Part model, mm, in its own coordinate system. Face numbers are marked on the shaded views. A direction names the side the tool comes from. Round coordinates to 2 decimals unless told otherwise and drop trailing zeros. Write each loop counter-clockwise with the first axis right and the second up, starting at its lowest first coordinate (ties: lowest second). Pieces come first, ordered by that corner, then holes. Notation, with made-up numbers: (28.5, 49) -> (37.5, 49) arc R19 ccw to (37.5, 83) -> close; hole circle Ø2 at (-17.5, 57). An arc over 180 degrees is marked (long way). Use CSV: the item, a comma, the result in double quotes. Start each with the question number.
(1) Probe line 1 (Y direction, x = -10.5, z = 0.45); line 2 (X direction, y = -1.5, z = 3.5); line 3 (Z direction, x = -9, y = 4). List the from-to ranges inside material, lowest first. Write a range as [from, to].
(2) Drop flat-ended pins along their axis: pin 1 (4 mm diameter, centred on x = -7, z = 2, fed in from +Y); pin 2 (2.5 mm diameter, centred on y = -1, z = 2.5, fed in from -X); pin 3 (1 mm diameter, centred on x = -11.5, y = -3, fed in from +Z); pin 4 (8 mm diameter, centred on x = -2, z = 12.5, fed in from +Y). Give the stop position or say it passes through.
(3) Saw through at B-B (z = 7). Give the cut face in (x, y).
(4) Which spindle directions (+Z, -Z, +X, -X, +Y, -Y) get a long thin tool onto all of the face, cutting with end or side? Do the marked faces 4, 5, 6 and 7. Say none if no direction does.
(5) Two-plate mould, pull along Y, no slides. Class the marked faces 1, 2 and 3: released by +Y, released by -Y, zero draft, split by the parting line, or undercut.
(6) Saw through at A-A (x = 10.5). Count the separate pieces of the cut face and the enclosed holes in it, plus the area to 3 significant figures.
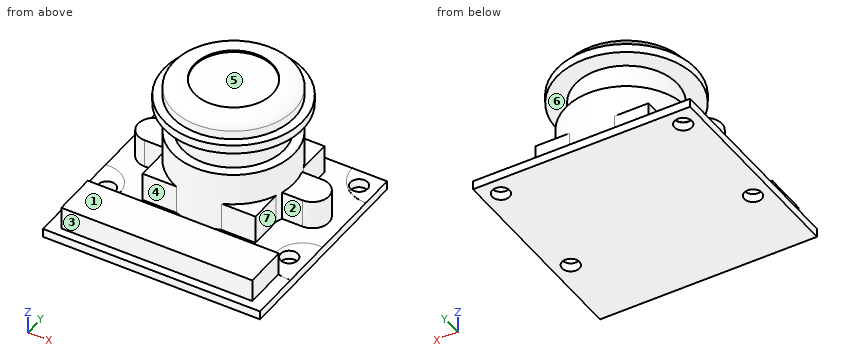
```python
from build123d import *

# Parameters (mm, degrees)
CROQUIS1_W              = 25
CROQUIS1_H              = 24
SALIENTE_EXTRUIR1_DEPTH = 1
CROQUIS2_W              = 22
CROQUIS2_H              = 5
SALIENTE_EXTRUIR2_DEPTH = 2.6
SALIENTE_EXTRUIR3_DEPTH = 3.3
CROQUIS5_R              = 7
SALIENTE_EXTRUIR4_DEPTH = 7
CROQUIS6_R              = 5.85
SALIENTE_EXTRUIR5_DEPTH = 3.5
CROQUIS9_R              = 1
CORTAR_EXTRUIR1_DEPTH   = 1
SALIENTE_EXTRUIR6_START = 0.01
CROQUIS10_R             = 0.972515087
CROQUIS10_R_2           = 1
SALIENTE_EXTRUIR6_DEPTH = 0.01


with BuildPart() as part:
    # Croquis1 → Saliente-Extruir1 (new body)
    with BuildSketch(Plane.XY):
        Rectangle(CROQUIS1_W, CROQUIS1_H)
    extrude(amount=SALIENTE_EXTRUIR1_DEPTH)

    # Croquis2 → Saliente-Extruir2 (add)
    with BuildSketch(Plane.XY.offset(1)):
        with Locations((0, -8.5)):
            Rectangle(CROQUIS2_W, CROQUIS2_H)
    extrude(amount=SALIENTE_EXTRUIR2_DEPTH)

    # Croquis3 → Saliente-Extruir3 (add)
    with BuildSketch(Plane.XY.offset(1)):
        with BuildLine():
            Line((-9.1, 5.4), (-6.5, 5.4))
            Line((-6.5, 5.4), (-6.5, 10))
            Line((-6.5, 10), (6.5, 10))
            Line((6.5, 10), (6.5, 5.4))
            Line((6.5, 5.4), (9.1, 5.4))
            ThreePointArc((9.1, 5.4), (11, 3.5), (9.1, 1.6))
            Line((9.1, 1.6), (6.5, 1.6))
            Line((6.5, 1.6), (6.5, -3))
            Line((6.5, -3), (-6.5, -3))
            Line((-6.5, -3), (-6.5, 1.6))
            Line((-6.5, 1.6), (-9.1, 1.6))
            ThreePointArc((-9.1, 1.6), (-11, 3.5), (-9.1, 5.4))
        make_face()
    extrude(amount=SALIENTE_EXTRUIR3_DEPTH)

    # Croquis5 → Saliente-Extruir4 (add)
    with BuildSketch(Plane.XY.offset(1)):
        with Locations(Location((0, 3.5, 0), (0, 0, 164.250707132))):
            Circle(CROQUIS5_R)
    extrude(amount=SALIENTE_EXTRUIR4_DEPTH)

    # Croquis6 → Saliente-Extruir5 (add)
    with BuildSketch(Plane.XY.offset(8)):
        with Locations((0, 3.5)):
            Circle(CROQUIS6_R)
    extrude(amount=SALIENTE_EXTRUIR5_DEPTH)

    # Croquis8 → Revolución1 (revolve)
    with BuildSketch(Plane(origin=(0, 3.5, 0), x_dir=(-1, 0, 0), z_dir=(0, -1, 0)), mode=Mode.PRIVATE) as revoluci_n1_sk:
        with BuildLine():
            Line((0, -11.5), (-8, -11.5))
            Line((-8, -11.5), (-8, -12.5))
            Line((-8, -12.5), (-7, -12.5))
            Line((-7, -12.5), (-7, -13.5))
            add(Edge.make_bspline(
                [(-7, -13.5), (-7, -14.5), (-4.5, -14.5)],
                knots=[0, 0, 0, 1.570796327, 1.570796327, 1.570796327], degree=2, weights=[1, 0.707106781, 1]))
            Line((-4.5, -14.5), (-4.5, -14.3))
            Line((-4.5, -14.3), (0, -14.3))
            Line((0, -14.3), (0, -11.5))
        make_face()
    revolve(revoluci_n1_sk.sketch.rotate(Axis((0, 3.5, 11.5), (0, 0, 1)), 180), axis=Axis((0, 3.5, 11.5), (0, 0, 1)))

    # Croquis9 → Cortar-Extruir1 (cut)
    with BuildSketch(Plane.XY.offset(1)):
        with Locations((-10.5, 10)):
            Circle(CROQUIS9_R)
        with Locations((-10.5, -3.2)):
            Circle(CROQUIS9_R)
        with Locations((10.5, -3.2)):
            Circle(CROQUIS9_R)
        with Locations((10.5, 10)):
            Circle(CROQUIS9_R)
    extrude(amount=-CORTAR_EXTRUIR1_DEPTH, mode=Mode.SUBTRACT)

    # Croquis10 → Saliente-Extruir6 (add)
    # profile 1 of 4: a face of its own
    with BuildSketch(Plane.XY.offset(1).offset(SALIENTE_EXTRUIR6_START)):
        with BuildLine():
            Line((-12.5, 8), (-12.5, 12))
            Line((-12.5, 12), (-8.5, 12))
            ThreePointArc((-8.5, 12), (-9.671572875, 9.171572875), (-12.5, 8))
        make_face()
        with Locations(Location((-10.5, 10, 0), (0, 0, 180))):
            Circle(CROQUIS10_R, mode=Mode.SUBTRACT)
    # profile 2 of 4: a face of its own
    with BuildSketch(Plane.XY.offset(1).offset(SALIENTE_EXTRUIR6_START)):
        with BuildLine():
            Line((-12.5, -0.2), (-12.5, -6.2))
            ThreePointArc((-12.5, -6.2), (-9, -3.2), (-12.5, -0.2))
        make_face()
        with Locations((-10.5, -3.2)):
            Circle(CROQUIS10_R_2, mode=Mode.SUBTRACT)
    # profile 3 of 4: a face of its own
    with BuildSketch(Plane.XY.offset(1).offset(SALIENTE_EXTRUIR6_START)):
        with BuildLine():
            Line((8.5, 12), (12.5, 12))
            Line((12.5, 12), (12.5, 8))
            ThreePointArc((12.5, 8), (9.671572875, 9.171572875), (8.5, 12))
        make_face()
        with Locations((10.5, 10)):
            Circle(CROQUIS10_R_2, mode=Mode.SUBTRACT)
    # profile 4 of 4: a face of its own
    with BuildSketch(Plane.XY.offset(1).offset(SALIENTE_EXTRUIR6_START)):
        with BuildLine():
            Line((12.5, -6.2), (12.5, -0.2))
            ThreePointArc((12.5, -0.2), (9, -3.2), (12.5, -6.2))
        make_face()
        with Locations((10.5, -3.2)):
            Circle(CROQUIS10_R_2, mode=Mode.SUBTRACT)
    extrude(amount=-SALIENTE_EXTRUIR6_DEPTH)


solid = part.part
```
Answers:
1,line 1,"y = [-12, -4.2], [-2.2, 9], [11, 12]"
1,line 2,"x = [-6.5, 6.5]"
1,line 3,"z = [0, 4.3]"
2,pin 1,"stops at y = 12"
2,pin 2,"stops at x = -6.5"
2,pin 3,"stops at z = 1.01"
2,pin 4,"stops at y = 11.5"
3,outline,"circle Ø14 at (0, 3.5)"
4,face 4,"-X"
4,face 5,"+Z"
4,face 6,"none"
4,face 7,"+X"
5,face 1,"zero draft"
5,face 2,"undercut"
5,face 3,"released by -Y"
6,separate pieces,"3"
6,enclosed holes,"0"
6,area,"41.5 mm²"
